Read the model definition and answer for the solid it produces. Units are mm, in the model's axes. Coordinates: 2 decimals unless noted, no trailing zeros. Write each loop counter-clockwise with the first axis right and the second up, starting at its lowest first coordinate (ties: lowest second). Pieces come first, ordered by that corner, then holes. Notation, with made-up numbers: M 67,65.25 L 109,65.25 A32 ccw 109,104.25 Z; hole C -6.5,88.5 d3. An arc over 180 degrees is marked long. Write item = value, one per line.
from build123d import *

# Parameters (mm, degrees)
RESSALTO_EXTRUS_O1_DEPTH = 75
CHANFRO1_SIZE            = 0.2
ESBO_O2_R                = 2.1
CORTE_EXTRUS_O1_DEPTH    = 150


with BuildPart() as part:
    # Esboço1 → Ressalto-extrusão1 (new body, symmetric)
    with BuildSketch(Plane(origin=(0, 0, 0), x_dir=(0, 0, -1), z_dir=(1, 0, 0))):
        with BuildLine():
            Line((-3.5, 0), (3.5, 0))
            Line((3.5, 0), (3.5, 2.5))
            ThreePointArc((3.5, 2.5), (2.7, 3.3), (3.5, 4.1))
            Line((3.5, 4.1), (3.5, 4.8))
            Line((3.5, 4.8), (-3.5, 4.8))
            Line((-3.5, 4.8), (-3.5, 4.1))
            ThreePointArc((-3.5, 4.1), (-2.7, 3.3), (-3.5, 2.5))
            Line((-3.5, 2.5), (-3.5, 0))
        make_face()
    extrude(amount=RESSALTO_EXTRUS_O1_DEPTH, both=True)

    # Chanfro1
    chanfro1_edges = [part.edges().sort_by_distance(p)[0] for p in [
        (0, 0, -3.5),
        (0, 0, 3.5),
        (0, 4.8, 3.5),
        (0, 4.8, -3.5),
    ]]
    chamfer(chanfro1_edges, length=CHANFRO1_SIZE)

    # Esboço2 → Corte-extrusão1 (cut)
    with BuildSketch(Plane(origin=(0, 4.8, 0), x_dir=(1, 0, 0), z_dir=(0, 1, 0))):
        with Locations((-7.5, 0)):
            Circle(ESBO_O2_R)
        with Locations((-22.5, 0)):
            Circle(ESBO_O2_R)
        with Locations((-37.5, 0)):
            Circle(ESBO_O2_R)
        with Locations((-52.5, 0)):
            Circle(ESBO_O2_R)
        with Locations((-67.5, 0)):
            Circle(ESBO_O2_R)
        with Locations((67.5, 0)):
            Circle(ESBO_O2_R)
        with Locations((52.5, 0)):
            Circle(ESBO_O2_R)
        with Locations((37.5, 0)):
            Circle(ESBO_O2_R)
        with Locations((22.5, 0)):
            Circle(ESBO_O2_R)
        with Locations((7.5, 0)):
            Circle(ESBO_O2_R)
    extrude(amount=-CORTE_EXTRUS_O1_DEPTH, mode=Mode.SUBTRACT)


solid = part.part
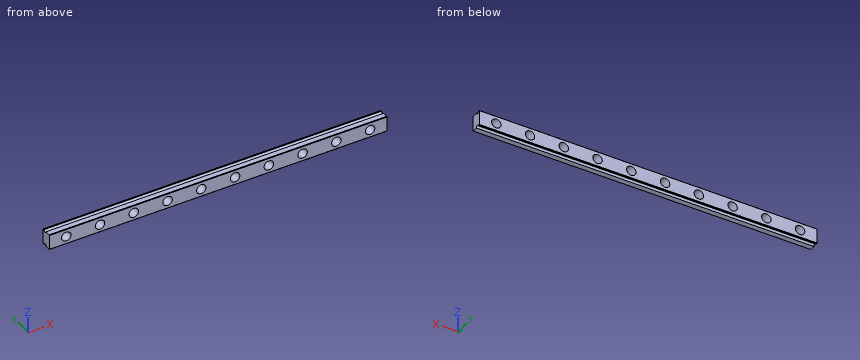
Item 1: Find section D-D (x = 58). Determine the outline of the cut face in (y, z), and give its area (3 significant figures).
Worked answers:
outline = M 0,-3.3 L 0.2,-3.5 L 2.5,-3.5 A0.8 cw 4.1,-3.5 L 4.6,-3.5 L 4.8,-3.3 L 4.8,3.3 L 4.6,3.5 L 4.1,3.5 A0.8 cw 2.5,3.5 L 0.2,3.5 L 0,3.3 Z
area = 31.5 mm²
Item 2: Consider line 1 along Z through (x, y) = (-22.5, 3.45); line 2 along Z through (x, y) = (7.5, 1.95); line 3 along Y through (x, z) = (-56, -3). Determine where each line is inside the solid, lowest interval first. Write a range as from..to.
Worked answers:
line_1 = -2.71..-2.1, 2.1..2.71
line_2 = -3.5..-2.1, 2.1..3.5
line_3 = 0..2.68, 3.92..4.8
Item 3: Find section A-A (x = -37.5). Determine the outline of the cut face in (y, z), and give its area (3 significant figures).
Worked answers:
outline = M 0,-3.3 L 0.2,-3.5 L 2.5,-3.5 A0.8 cw 4.1,-3.5 L 4.6,-3.5 L 4.8,-3.3 L 4.8,-2.1 L 0,-2.1 Z; M 0,2.1 L 4.8,2.1 L 4.8,3.3 L 4.6,3.5 L 4.1,3.5 A0.8 cw 2.5,3.5 L 0.2,3.5 L 0,3.3 Z
area = 11.3 mm²
Item 4: Find section B-B (y = 1). State how many separate pieces and enclosed holes the cut face has, and give its area (3 significant figures).
Worked answers:
separate_pieces = 1
enclosed_holes = 10
area = 911 mm²
